Design review of the part built by this model. Coordinates are the model's own, in mm. A direction names the side the tool comes from. Coordinates: 2 decimals unless noted, no trailing zeros. Loops run counter-clockwise (first coordinate to the right, second up) from the corner with the lowest first, then second, coordinate; pieces in that order, holes last. Notation, with made-up numbers: (10.5, 1) - (40.5, 1) arc R14 ccw to (40.5, 5) - close; hole circle Ø10 at (-26, 70.25). An arc over 180 degrees is marked (long way). Use one line per item in the form item = value. Start each with the question number.
(1) The part is to be moulded in two halves that separate along X. For faces 1 (the face through (24.1, 0.86, 2.54)), 2 (the face through (5.65, 21.49, 3.52)), 3 (the face through (12, 0, 2)), 4 (the face through (6, 17, 2)), say which applies: pulls with the +X half, pulls with the -X half, needs draft (parallel to the pull), parting line crosses it, or undercut.
(2) Tool access review of faces 5 (the face through (-2.819, 37, 5)), 6 (the face through (21, 2, 2)), 7 (the face through (12, 14, 5)), 8 (the face through (0, 16, 2)): name each direction out of +Z, -Z, +X, -X, +Y, -Y from which nothing blocks a thin tool from reaching the whole face with its end or side.
(3) Add section A-A (x = 20). State the section outline as (y, z) points.
(4) Add section B-B (z = 2.5). State the section outline as (x, y) points, plus the area to 3 significant figures.
(5) Clearance check with flat-ended pins moving along their axes: pin 1 Ø4 at (y, z) = (27.5, 1.5) entering from -X; pin 2 Ø6.5 at (x, y) = (21, 2.5) entering from +Z; pin 3 Ø5 at (y, z) = (31, 3) entering from -X; pin 4 Ø2 at (x, y) = (5, 18.56) entering from +Z. State where each tip first meets the part, or that it passes through.
(6) Add section C-C (y = 18). State the section outline as (x, z) points.
(7) For L1, parallel to Y at x = 5, z = 0.4; L2, parallel to Z at x = 3, y = 8.5; L3, parallel to Y at x = 10.5, z = 8.25, list the stretches that pass through material, from the lowest coordinate up.
(8) Add section D-D (z = 6.75). State the section outline as (x, y) points, plus the area to 3 significant figures.
```python
from build123d import *

# Parameters (mm, degrees)
F0_W     = 25
F0_H     = 30.0927665085
F0_W_2   = 30.6387297809
F0_H_2   = 5.7677225769
F1_DEPTH = 5
F2_R     = 1.675
F3_DEPTH = 25
F4_R     = 3
F5_DEPTH = 11
F6_R     = 1.4
F7_DEPTH = 11.001
F2_R_2   = 3
F8_DEPTH = 3
F9_R     = 3
F10_R    = 2


# Not quite as in the source:
# - a feature names something its author has since deleted; it is built from what else it names


with BuildPart() as f1:
    # F0 (on Top) → F1 (new body)
    with BuildSketch(Plane.XY):
        with Locations((12.5, 15.0463832542)):
            Rectangle(F0_W, F0_H)
        Polygon((-2.8193648905, 35.1040735841), (0, 30.0927665085), (25, 30.0927665085), (27.8193648905, 35.1040735841), align=None)
        with Locations((12.5, 37.9879348725)):
            Rectangle(F0_W_2, F0_H_2)
    extrude(amount=F1_DEPTH)

    # F2 (on face) → F3 (cut)
    with BuildSketch(Plane.XY.offset(5)):
        with BuildLine():
            ThreePointArc((3.325, 18.5605346784), (5, 16.8855346784), (6.675, 18.5605346784))
            ThreePointArc((6.675, 18.5605346784), (5, 20.2355346784), (3.325, 18.5605346784))
        make_face()
        with Locations((20, 18.5605346784)):
            Circle(F2_R)
        with Locations((20, 3.5605346784)):
            Circle(F2_R)
        with Locations((5, 3.5605346784)):
            Circle(F2_R)
    extrude(amount=-F3_DEPTH, mode=Mode.SUBTRACT)

    # F4
    f4_edges = [f1.edges().sort_by_distance(p)[0] for p in [
        (0, 0, 2.5),
        (25, 0, 2.5),
    ]]
    fillet(f4_edges, radius=F4_R)

    # F0 (on Top) → F5 (join)
    with BuildSketch(Plane.XY):
        with Locations((12.5, 37.9879348725)):
            Rectangle(F0_W_2, F0_H_2)
        Polygon((-2.8193648905, 35.1040735841), (0, 30.0927665085), (25, 30.0927665085), (27.8193648905, 35.1040735841), align=None)
    extrude(amount=F5_DEPTH)

    # F6 (on face) → F7 (cut, through all)
    with BuildSketch(Plane.XY.offset(11)):
        with Locations((23.6868802458, 37.1295362711)):
            Circle(F6_R)
        with BuildLine():
            ThreePointArc((-0.1581197542, 37.1295362711), (1.2418802458, 35.7295362711), (2.6418802458, 37.1295362711))
            ThreePointArc((2.6418802458, 37.1295362711), (1.2418802458, 38.5295362711), (-0.1581197542, 37.1295362711))
        make_face()
    extrude(amount=-F7_DEPTH, mode=Mode.SUBTRACT)

    # F2 (on face) → F8 (cut)
    with BuildSketch(Plane.XY.offset(5)):
        with BuildLine():
            ThreePointArc((8, 18.5605346784), (5, 21.5605346784), (2, 18.5605346784))
            ThreePointArc((2, 18.5605346784), (5, 15.5605346784), (8, 18.5605346784))
        make_face()
        with BuildLine():
            ThreePointArc((3.325, 18.5605346784), (5, 20.2355346784), (6.675, 18.5605346784))
            ThreePointArc((6.675, 18.5605346784), (5, 16.8855346784), (3.325, 18.5605346784))
        make_face(mode=Mode.SUBTRACT)
        with Locations((5, 3.5605346784)):
            Circle(F2_R_2)
        with Locations((5, 3.5605346784)):
            Circle(F2_R, mode=Mode.SUBTRACT)
        with Locations((20, 18.5605346784)):
            Circle(F2_R_2)
        with Locations((20, 18.5605346784)):
            Circle(F2_R, mode=Mode.SUBTRACT)
        with Locations((20, 3.5605346784)):
            Circle(F2_R_2)
        with Locations((20, 3.5605346784)):
            Circle(F2_R, mode=Mode.SUBTRACT)
    extrude(amount=-F8_DEPTH, mode=Mode.SUBTRACT)

    # F9
    f9_edges = [f1.edges().sort_by_distance(p)[0] for p in [
        (12.5, 30.092767, 5),
    ]]
    fillet(f9_edges, radius=F9_R)

    # F10
    f10_edges = [f1.edges().sort_by_distance(p)[0] for p in [
        (27.819365, 40.871796, 5.5),
        (-2.819365, 40.871796, 5.5),
    ]]
    fillet(f10_edges, radius=F10_R)


solid = f1.part
```
Computed values:
q1.face_1 = pulls with the +X half
q1.face_2 = undercut
q1.face_3 = needs draft
q1.face_4 = undercut
q2.face_5 = +Z, -Z, -X, +Y, -Y
q2.face_6 = +Z
q2.face_7 = +Z, +X, -X, -Y
q2.face_8 = +Z, -Z, -X, -Y
q3.outline = (0, 0) - (1.89, 0) - (1.89, 2) - (0.56, 2) - (0.56, 5) - (0, 5) - close; (5.24, 0) - (16.89, 0) - (16.89, 2) - (15.56, 2) - (15.56, 5) - (6.56, 5) - (6.56, 2) - (5.24, 2) - close; (20.24, 0) - (40.87, 0) - (40.87, 11) - (30.09, 11) - (30.09, 8) arc R3 cw to (27.09, 5) - (21.56, 5) - (21.56, 2) - (20.24, 2) - close
q4.outline = (-2.82, 35.1) - (0, 30.09) - (0, 3) arc R3 ccw to (3, 0) - (22, 0) arc R3 ccw to (25, 3) - (25, 30.09) - (27.82, 35.1) - (27.82, 38.87) arc R2 ccw to (25.82, 40.87) - (-0.82, 40.87) arc R2 ccw to (-2.82, 38.87) - close; hole circle Ø2.8 at (1.24, 37.13); hole circle Ø6 at (5, 3.56); hole circle Ø6 at (5, 18.56); hole circle Ø6 at (20, 3.56); hole circle Ø6 at (20, 18.56); hole circle Ø2.8 at (23.69, 37.13)
q4.area = 937 mm^2
q5.pin_1 = 0
q5.pin_2 = 5
q5.pin_3 = -1.92
q5.pin_4 = through
q6.outline = (0, 0) - (3.42, 0) - (3.42, 2) - (2.05, 2) - (2.05, 5) - (0, 5) - close; (6.58, 0) - (18.42, 0) - (18.42, 2) - (17.05, 2) - (17.05, 5) - (7.95, 5) - (7.95, 2) - (6.58, 2) - close; (21.58, 0) - (25, 0) - (25, 5) - (22.95, 5) - (22.95, 2) - (21.58, 2) - close
q7.L1 = 0 to 1.89, 5.24 to 16.89, 20.24 to 40.87
q7.L2 = 0 to 5
q7.L3 = 30.09 to 40.87
q8.outline = (-2.82, 35.1) - (0, 30.09) - (0, 29.82) - (25, 29.82) - (25, 30.09) - (27.82, 35.1) - (27.82, 38.87) arc R2 ccw to (25.82, 40.87) - (-0.82, 40.87) arc R2 ccw to (-2.82, 38.87) - close; hole circle Ø2.8 at (1.24, 37.13); hole circle Ø2.8 at (23.69, 37.13)
q8.area = 309 mm^2
